CAD build for the part. Positions are in the model's coordinates, mm. Coordinates: 2 decimals unless noted, no trailing zeros. Write each loop counter-clockwise with the first axis right and the second up, starting at its lowest first coordinate (ties: lowest second). Pieces come first, ordered by that corner, then holes. Notation, with made-up numbers: (13.5, 22.5) - (21.5, 22.5) arc R23 cw to (21.5, 48.5) - close; hole circle Ø4 at (66, 52.5). An arc over 180 degrees is marked (long way). One line per question, with ' | ' between items. Start each with the question number.
1. Band-saw the part on B-B, the plane y = 256.5. Write the cut outline in (x, z), then the cut area to 3 significant figures.
2. Band-saw the part on A-A, the plane x = 36.5. Write the cut outline in (y, z), then the cut area to 3 significant figures.
3. Two-plate mould, pull along X, no slides. Class faces 1 (the flat face through (51, 253, 0)), 2 (the cylindrical face through (40.63, 286.91, 0.74)): +X half, -X half, draft (parallel to the pull), parting line (faces both ways), or undercut.
4. Flat gauge pins, fed straight in: P1, Ø0.8, axis at y = 242, z = 1, coming from the -X side; P2, Ø0.8, axis at x = 63.5, z = 1, coming from the -Y side. Where does each tip first touch, or does it go through?
5. Band-saw the part on D-D, the plane y = 272. Write the cut outline in (x, z), then the cut area to 3 significant figures.
6. Probe line 1 (Y direction, x = 38, z = 0.6); line 2 (X direction, y = 274, z = 1.3); line 3 (X direction, y = 247, z = 0.95). List the from-to ranges inside material, lowest first.
7. Band-saw the part on C-C, the plane x = 29.5. Write the cut outline in (y, z).
from build123d import *

# Parameters (mm, degrees)
MODEL_R                 = 29
MODEL_R_2               = 16.5
SALIENTE_EXTRUIR1_DEPTH = 1.5


with BuildPart() as part:
    # Model → Saliente-Extruir1 (new body)
    with BuildSketch(Plane.XY):
        with Locations((38.490393449, 265.517783021)):
            Circle(MODEL_R)
        with Locations((38.490393449, 265.517783021)):
            Circle(MODEL_R_2, mode=Mode.SUBTRACT)
        with BuildLine():
            Line((38.490393449, 287.017783021), (38.490393449, 292.767783021))
            ThreePointArc((38.490393449, 292.767783021), (41.161360523, 292.636566823), (43.806604724, 292.244181912))
            Line((43.806604724, 292.244181912), (42.684835372, 286.60466655))
            ThreePointArc((42.684835372, 286.60466655), (40.597761966, 286.914254645), (38.490393449, 287.017783021))
        make_face(mode=Mode.SUBTRACT)
        with BuildLine():
            Line((34.295951526, 286.60466655), (33.174182174, 292.244181912))
            ThreePointArc((33.174182174, 292.244181912), (30.580135994, 291.59440717), (28.062269917, 290.693500282))
            Line((28.062269917, 290.693500282), (30.262699653, 285.38119297))
            ThreePointArc((30.262699653, 285.38119297), (32.249272888, 286.09200024), (34.295951526, 286.60466655))
        make_face(mode=Mode.SUBTRACT)
        with BuildLine():
            Line((26.545633439, 283.394379686), (23.351104599, 288.175329957))
            ThreePointArc((23.351104599, 288.175329957), (21.203176455, 286.582317876), (19.221733662, 284.786442809))
            Line((19.221733662, 284.786442809), (23.287597653, 280.720578817))
            ThreePointArc((23.287597653, 280.720578817), (24.850937839, 282.137507769), (26.545633439, 283.394379686))
        make_face(mode=Mode.SUBTRACT)
        with BuildLine():
            Line((20.613796784, 277.462543031), (15.832846514, 280.657071871))
            ThreePointArc((15.832846514, 280.657071871), (14.458038995, 278.3633441), (13.314676188, 275.945906553))
            Line((13.314676188, 275.945906553), (18.6269835, 273.745476817))
            ThreePointArc((18.6269835, 273.745476817), (19.529086265, 275.652812863), (20.613796784, 277.462543031))
        make_face(mode=Mode.SUBTRACT)
        with BuildLine():
            Line((17.40350992, 269.712224945), (11.763994558, 270.833994296))
            ThreePointArc((11.763994558, 270.833994296), (11.371609647, 268.188750095), (11.240393449, 265.517783021))
            Line((11.240393449, 265.517783021), (16.990393449, 265.517783021))
            ThreePointArc((16.990393449, 265.517783021), (17.093921825, 267.625151538), (17.40350992, 269.712224945))
        make_face(mode=Mode.SUBTRACT)
        with BuildLine():
            Line((17.40350992, 261.323341098), (11.763994558, 260.201571746))
            ThreePointArc((11.763994558, 260.201571746), (12.4137693, 257.607525566), (13.314676188, 255.089659489))
            Line((13.314676188, 255.089659489), (18.6269835, 257.290089226))
            ThreePointArc((18.6269835, 257.290089226), (17.916176231, 259.27666246), (17.40350992, 261.323341098))
        make_face(mode=Mode.SUBTRACT)
        with BuildLine():
            Line((20.613796784, 253.573023011), (15.832846514, 250.378494172))
            ThreePointArc((15.832846514, 250.378494172), (17.425858595, 248.230566028), (19.221733662, 246.249123234))
            Line((19.221733662, 246.249123234), (23.287597653, 250.314987226))
            ThreePointArc((23.287597653, 250.314987226), (21.870668702, 251.878327412), (20.613796784, 253.573023011))
        make_face(mode=Mode.SUBTRACT)
        with BuildLine():
            Line((26.545633439, 247.641186357), (23.351104599, 242.860236086))
            ThreePointArc((23.351104599, 242.860236086), (25.64483237, 241.485428568), (28.062269917, 240.34206576))
            Line((28.062269917, 240.34206576), (30.262699653, 245.654373072))
            ThreePointArc((30.262699653, 245.654373072), (28.355363607, 246.556475838), (26.545633439, 247.641186357))
        make_face(mode=Mode.SUBTRACT)
        with BuildLine():
            Line((34.295951526, 244.430899493), (33.174182174, 238.79138413))
            ThreePointArc((33.174182174, 238.79138413), (35.819426375, 238.39899922), (38.490393449, 238.267783021))
            Line((38.490393449, 238.267783021), (38.490393449, 244.017783021))
            ThreePointArc((38.490393449, 244.017783021), (36.383024932, 244.121311398), (34.295951526, 244.430899493))
        make_face(mode=Mode.SUBTRACT)
        with BuildLine():
            Line((42.684835372, 244.430899493), (43.806604724, 238.79138413))
            ThreePointArc((43.806604724, 238.79138413), (46.400650904, 239.441158873), (48.918516981, 240.34206576))
            Line((48.918516981, 240.34206576), (46.718087245, 245.654373072))
            ThreePointArc((46.718087245, 245.654373072), (44.73151401, 244.943565803), (42.684835372, 244.430899493))
        make_face(mode=Mode.SUBTRACT)
        with BuildLine():
            Line((50.435153459, 247.641186357), (53.629682299, 242.860236086))
            ThreePointArc((53.629682299, 242.860236086), (55.777610442, 244.453248167), (57.759053236, 246.249123234))
            Line((57.759053236, 246.249123234), (53.693189244, 250.314987226))
            ThreePointArc((53.693189244, 250.314987226), (52.129849058, 248.898058274), (50.435153459, 247.641186357))
        make_face(mode=Mode.SUBTRACT)
        with BuildLine():
            Line((56.366990113, 253.573023011), (61.147940384, 250.378494172))
            ThreePointArc((61.147940384, 250.378494172), (62.522747902, 252.672221943), (63.66611071, 255.089659489))
            Line((63.66611071, 255.089659489), (58.353803398, 257.290089226))
            ThreePointArc((58.353803398, 257.290089226), (57.451700632, 255.38275318), (56.366990113, 253.573023011))
        make_face(mode=Mode.SUBTRACT)
        with BuildLine():
            Line((59.577276978, 261.323341098), (65.21679234, 260.201571746))
            ThreePointArc((65.21679234, 260.201571746), (65.609177251, 262.846815947), (65.740393449, 265.517783021))
            Line((65.740393449, 265.517783021), (59.990393449, 265.517783021))
            ThreePointArc((59.990393449, 265.517783021), (59.886865072, 263.410414504), (59.577276978, 261.323341098))
        make_face(mode=Mode.SUBTRACT)
        with BuildLine():
            Line((59.577276978, 269.712224945), (65.21679234, 270.833994296))
            ThreePointArc((65.21679234, 270.833994296), (64.567017598, 273.428040477), (63.66611071, 275.945906553))
            Line((63.66611071, 275.945906553), (58.353803398, 273.745476817))
            ThreePointArc((58.353803398, 273.745476817), (59.064610667, 271.758903582), (59.577276978, 269.712224945))
        make_face(mode=Mode.SUBTRACT)
        with BuildLine():
            Line((56.366990113, 277.462543031), (61.147940384, 280.657071871))
            ThreePointArc((61.147940384, 280.657071871), (59.554928303, 282.805000015), (57.759053236, 284.786442809))
            Line((57.759053236, 284.786442809), (53.693189244, 280.720578817))
            ThreePointArc((53.693189244, 280.720578817), (55.110118196, 279.157238631), (56.366990113, 277.462543031))
        make_face(mode=Mode.SUBTRACT)
        with BuildLine():
            Line((50.435153459, 283.394379686), (53.629682299, 288.175329957))
            ThreePointArc((53.629682299, 288.175329957), (51.335954527, 289.550137475), (48.918516981, 290.693500282))
            Line((48.918516981, 290.693500282), (46.718087245, 285.38119297))
            ThreePointArc((46.718087245, 285.38119297), (48.625423291, 284.479090205), (50.435153459, 283.394379686))
        make_face(mode=Mode.SUBTRACT)
    extrude(amount=SALIENTE_EXTRUIR1_DEPTH)


solid = part.part
Filled in:
1) outline: (10.93, 0) - (12.78, 0) - (12.78, 1.5) - (10.93, 1.5) - close; (16.72, 0) - (24.67, 0) - (24.67, 1.5) - (16.72, 1.5) - close; (52.31, 0) - (58.01, 0) - (58.01, 1.5) - (52.31, 1.5) - close; (60.26, 0) - (66.05, 0) - (66.05, 1.5) - (60.26, 1.5) - close | area: 31.9 mm²
2) outline: (236.59, 0) - (238.34, 0) - (238.34, 1.5) - (236.59, 1.5) - close; (244.11, 0) - (249.14, 0) - (249.14, 1.5) - (244.11, 1.5) - close; (281.9, 0) - (294.45, 0) - (294.45, 1.5) - (281.9, 1.5) - close | area: 29.0 mm²
3) face 1: draft | face 2: undercut
4) P1: stops at x = 20.98 | P2: stops at y = 250.18
5) outline: (10.22, 0) - (23.32, 0) - (23.32, 1.5) - (10.22, 1.5) - close; (53.66, 0) - (58.99, 0) - (58.99, 1.5) - (53.66, 1.5) - close; (64.96, 0) - (66.76, 0) - (66.76, 1.5) - (64.96, 1.5) - close | area: 30.3 mm²
6) line 1: y = 236.52 to 238.27, 244.02 to 249.03, 282.01 to 294.51 | line 2: x = 10.76 to 18.01, 18.73 to 24.34, 52.64 to 58.97, 64.39 to 66.22 | line 3: x = 16.17 to 18.5, 19.97 to 26.12, 27.57 to 50.86, 57.01 to 60.81
7) outline: (237.95, 0) - (243.81, 0) - (243.81, 1.5) - (237.95, 1.5) - close; (245.99, 0) - (251.68, 0) - (251.68, 1.5) - (245.99, 1.5) - close; (279.35, 0) - (287.22, 0) - (287.22, 1.5) - (279.35, 1.5) - close; (291.24, 0) - (293.09, 0) - (293.09, 1.5) - (291.24, 1.5) - close
